Autodesk Inventor part; units mm, degrees
ref_plane "YZ Plane" through (0, 0, 0) normal (1, 0, 0) x (0, 1, 0)
ref_plane "XZ Plane" through (0, 0, 0) normal (0, 1, 0) x (-1, 0, 0)
ref_plane "XY Plane" through (0, 0, 0) normal (0, 0, 1) x (1, 0, 0)
sketch "Эскиз1" plane through (0, 0, 0) normal (0, 0, 1) x (1, 0, 0)
  line L0 (4.4225, 1.3322) -> (3.365, -3.1639)
  line L1 (3.365, -3.1639) -> (-1.0575, -4.4961)
  line L2 (-1.0575, -4.4961) -> (-4.4225, -1.3322)
  line L3 (-4.4225, -1.3322) -> (-3.365, 3.1639)
  line L4 (-3.365, 3.1639) -> (1.0575, 4.4961)
  line L5 (1.0575, 4.4961) -> (4.4225, 1.3322)
  circle A0 centre (0, 0) radius 2
  point P0 (-1.1537, 3.83)
  dimension "d0" = 8
  dimension "d1" = 7.66
  dimension "d2" = 4
extrude "Выдавливание1" add sketch "Эскиз1" along normal blind 65
properties part number "стойка"
Input: part model. Units: mm. Frame: model coordinates. Coordinates: 2 decimals unless noted, no trailing zeros. Loops run counter-clockwise (first coordinate to the right, second up) from the corner with the lowest first, then second, coordinate; pieces in that order, holes last. Notation, with made-up numbers: M 76,-11.75 L 135,-11.75 A37 ccw 135,25.25 Z; hole C 73,67 d3. An arc over 180 degrees is marked long. One line per item, written item: value.
(1) Section C-C (y = 0). Output: boundary loops of the cut face in (x, z).
Filled in:
outline: M -4.11,0 L -2,0 L -2,65 L -4.11,65 Z; M 2,0 L 4.11,0 L 4.11,65 L 2,65 Z
(2) Line query: line 1 along Y through (x, z) = (0, 31); line 2 along X through (y, z) = (0.25, 50); line 3 along X through (y, z) = (-1, 57.5). Output: solid intervals per line, ascending. Write a range as from..to.
Filled in:
line 1: -4.18..-2, 2..4.18
line 2: -4.05..-1.98, 1.98..4.17
line 3: -4.34..-1.73, 1.73..3.87
(3) Section B-B (x = 0). Output: boundary loops of the cut face in (y, z).
Filled in:
outline: M -4.18,0 L -2,0 L -2,65 L -4.18,65 Z; M 2,0 L 4.18,0 L 4.18,65 L 2,65 Z
(4) Section A-A (z = 17). Output: boundary loops of the cut face in (x, y) (1 decimal), and give its area (3 significant figures).
Filled in:
outline: M -4.4,-1.3 L -1.1,-4.5 L 3.4,-3.2 L 4.4,1.3 L 1.1,4.5 L -3.4,3.2 Z; hole C 0,0 d4
area: 42.9 mm^2
(5) Pull-direction query (Y, two-part tool) for faces 1 (the cylindrical face through (0, 2, 32)), 2 (the flat face through (-1.185, 3.821, 32.045)), 3 (the flat face through (2, 1, 0)); classes: +Y half, -Y half, draft (parallel to the pull), parting line (faces both ways), or undercut.
Filled in:
face 1: undercut
face 2: +Y half
face 3: draft
